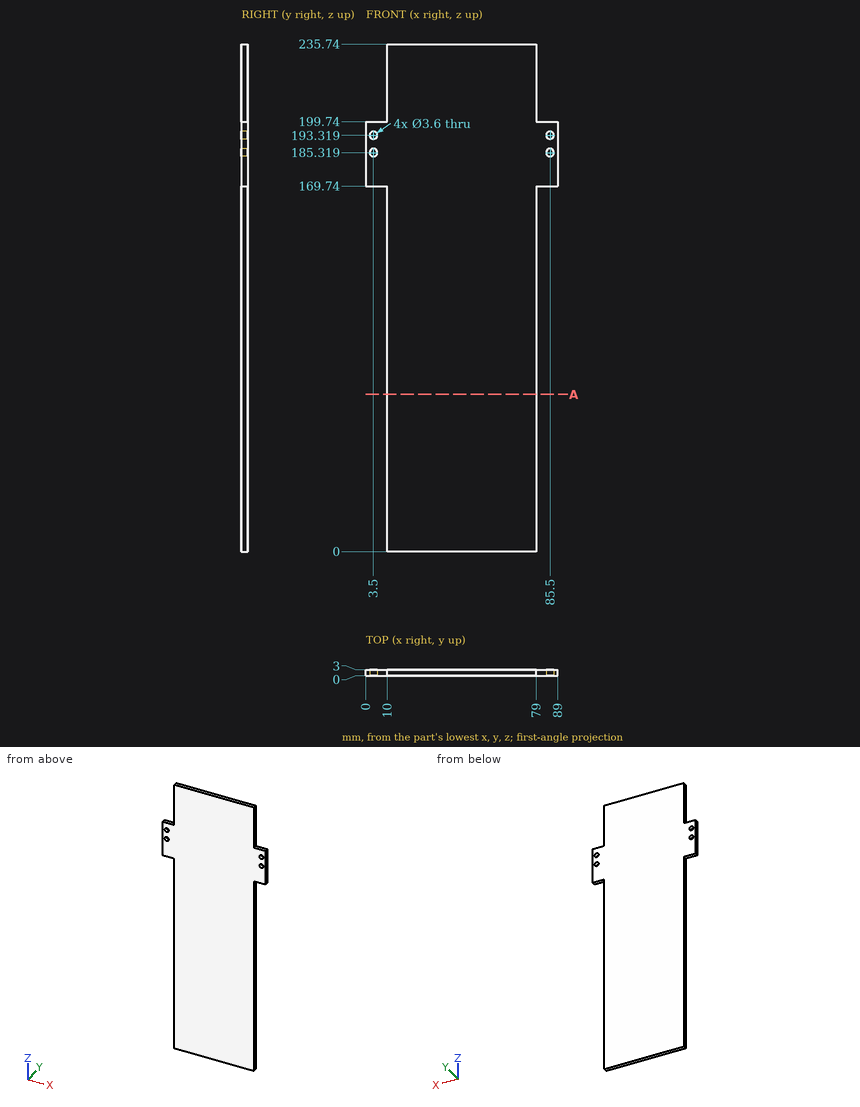
Job drawing, mm, ordinate dimensions from the low corner. One solid piece. Round coordinates to 2 decimals unless told otherwise and drop trailing zeros. Write each loop counter-clockwise with the first axis right and the second up, starting at its lowest first coordinate (ties: lowest second). Pieces come first, ordered by that corner, then holes.
1) Pin check, flat tips, straight feed: pin 1 (1.5 mm diameter, centred on y = 1, z = 223.5, fed in from -X); pin 2 (1.5 mm diameter, centred on y = 1, z = 51, fed in from +X); pin 3 (3 mm diameter, centred on x = 3.5, z = 185.32, fed in from +Y); pin 4 (0.9 mm diameter, centred on x = 84.5, y = 1.5, fed in from +Z). Stop position of each tip, or through.
2) Band-saw the part on A-A, the plane z = 73. List the corners of the cut face in (x, y), and give its area (3 significant figures).
3) Drill centre lines: probe 1 along Z at (x, y) = (3.5, 1.5); probe 2 along X at (y, z) = (2.55, 25.5). Where is each one in solid material? Low to high.
Ans:
1. pin 1: stops at x = 10
1. pin 2: stops at x = 79
1. pin 3: passes through
1. pin 4: stops at z = 199.74
2. outline: (10, 0) - (79, 0) - (79, 3) - (10, 3) - close
2. area: 207 mm2
3. probe 1: z = 169.74 to 183.52, 187.12 to 191.52, 195.12 to 199.74
3. probe 2: x = 10 to 79
